from build123d import *

# Parameters (mm, degrees)
F0_W     = 140
F0_H     = 59
F1_DEPTH = 3
F2_R     = 1.5
F3_DEPTH = 25
F4_SIZE  = 2


with BuildPart() as f1:
    # F0 (on Front) → F1 (new body)
    with BuildSketch(Plane.XZ):
        Rectangle(F0_W, F0_H)
        Polygon((85, -29.5), (70, 29.5), (70, -29.5), align=None)
    extrude(amount=F1_DEPTH)

    # F2 (on face) → F3 (cut)
    with BuildSketch(Plane.XZ.offset(3)):
        with Locations((-60, 14)):
            Circle(F2_R)
        with Locations((60, 14)):
            Circle(F2_R)
        with Locations((60, -14)):
            Circle(F2_R)
        with Locations((-60, -14)):
            Circle(F2_R)
    extrude(amount=-F3_DEPTH, mode=Mode.SUBTRACT)

    # F4
    f4_edges = [f1.edges().sort_by_distance(p)[0] for p in [
        (-61.5, 0, -14),
        (-61.5, 0, 14),
        (58.5, 0, -14),
        (58.5, 0, 14),
    ]]
    chamfer(f4_edges, length=F4_SIZE)


solid = f1.part
Here's how the part is built. I have some questions about the finished solid (model axes, mm). Give positions to 0.01 mm unless a question says otherwise; leave off trailing zeros. Order: outer loops, then holes, each group sorted by start corner. A loop starts at its lowest first (then second) coordinate and runs counter-clockwise, first axis right, second up. Notation, with made-up numbers: (85.25, 38) -> (107.25, 38) arc R26 cw to (107.25, 58) -> close; hole circle Ø3 at (36.25, 4.25). An arc over 180 degrees is marked (long way). Use a Markdown table: item, result. Add a question column.
Item 1: I need wall thicknesses on line 1 (Z direction, x = 60, y = -2.4); line 2 (X direction, y = -0.2, z = 15.5); line 3 (X direction, y = -2.35, z = -24.5). Which ranges of each line are inside material? Lowest first, please.
Item 2: Will these pins go through, and if not, where does the flat tip stop? pin 1 (5 mm diameter, centred on x = 60, z = -14, fed in from +Y); pin 2 (1 mm diameter, centred on y = -1.5, z = -11.5, fed in from +X); pin 3 (4 mm diameter, centred on x = 60, z = 14, fed in from +Y).
Item 3: Imagine slicing it at B-B on z = -14. Please give me the cut outline in (x, y), plus the area to 3 significant figures.
Item 4: Imagine slicing it at A-A on x = 60. Please give me the cut outline in (y, z).
Item 5: Imagine slicing it at C-C on z = 23. Please give me the cut outline in (x, y).
Item 6: If we mould it in two halves opening along Z, with no side actions, what happens to faces 1 (the face through (-1, -1, 29.5)), 2 (the face through (-58.57, -2.51, -13.55)), 3 (the face through (6, 0, 0))? For each: pulls with the +Z half, pulls with the -Z half, needs draft (parallel to the pull), parting line crosses it, or undercut.
Data:
| question | item | result |
|---|---|---|
| 1 | line 1 | z = -29.5 to -15.5, -12.5 to 12.5, 15.5 to 29.5 |
| 1 | line 2 | x = -70 to -62.94, -57.06 to 57.06, 62.94 to 73.56 |
| 1 | line 3 | x = -70 to 83.73 |
| 2 | pin 1 | stops at y = -1 |
| 2 | pin 2 | stops at x = 80.55 |
| 2 | pin 3 | stops at y = -1.5 |
| 3 | outline | (-70, -3) -> (-61.5, -3) -> (-61.5, -2) -> (-63.5, 0) -> (-70, 0) -> close; (-58.5, -3) -> (58.5, -3) -> (58.5, -2) -> (56.5, 0) -> (-56.5, 0) -> (-58.5, -2) -> close; (61.5, -3) -> (81.06, -3) -> (81.06, 0) -> (63.5, 0) -> (61.5, -2) -> close |
| 3 | area | 427 mm² |
| 4 | outline | (-3, -29.5) -> (0, -29.5) -> (0, -17.5) -> (-2, -15.5) -> (-3, -15.5) -> close; (-3, -12.5) -> (-2, -12.5) -> (0, -10.5) -> (0, 10.5) -> (-2, 12.5) -> (-3, 12.5) -> close; (-3, 15.5) -> (-2, 15.5) -> (0, 17.5) -> (0, 29.5) -> (-3, 29.5) -> close |
| 5 | outline | (-70, -3) -> (71.65, -3) -> (71.65, 0) -> (-70, 0) -> close |
| 6 | face 1 | pulls with the +Z half |
| 6 | face 2 | undercut |
| 6 | face 3 | needs draft |
